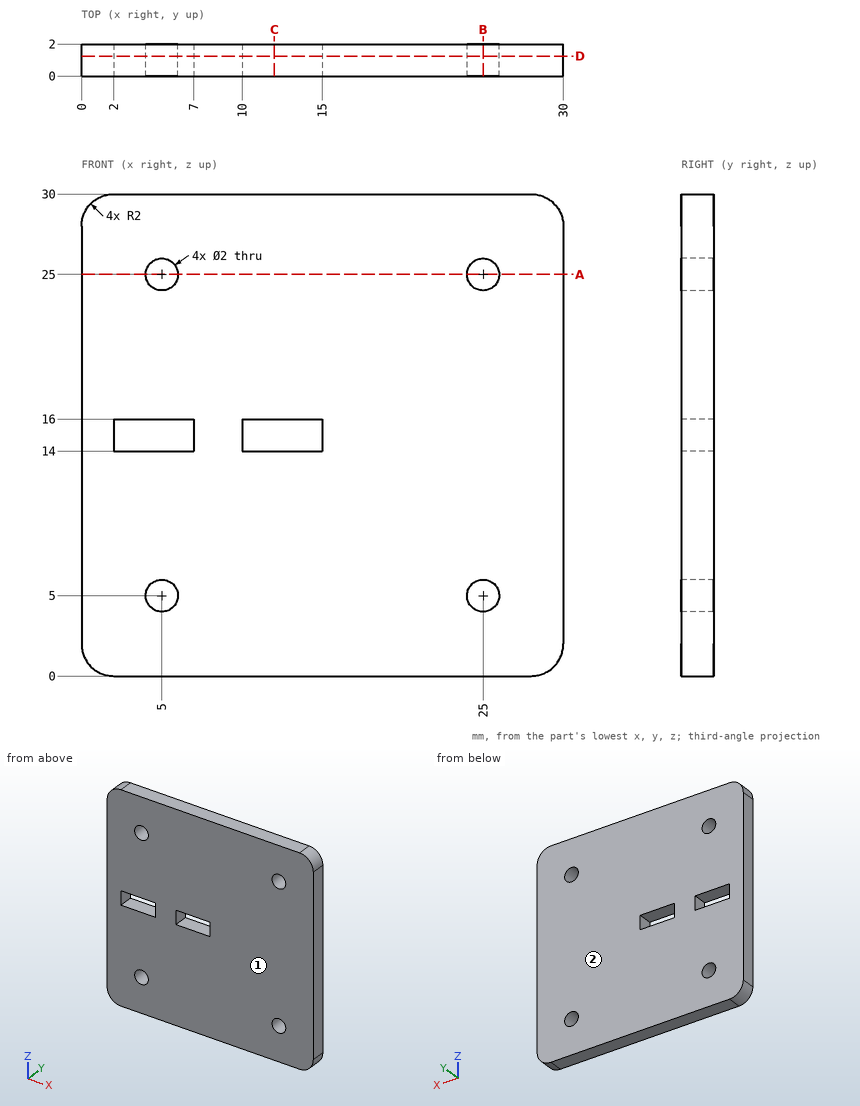
Geometry check sheet. Reference: drawing and pictorial views, mm from the part's lowest x, y, z. Round coordinates to 2 decimals unless told otherwise and drop trailing zeros. Order: outer loops, then holes, each group sorted by start corner. A loop starts at its lowest first (then second) coordinate and runs counter-clockwise, first axis right, second up. Notation, with made-up numbers: M -29.75,-4.5 L 18.25,-4.5 A19 ccw 18.25,15.5 Z; hole C -7,69.25 d1. An arc over 180 degrees is marked long. Answer as CSV lines item,"result".
1) Sectioned sample at A-A on z = 25. Record the cut outline in (x, y).
Entries:
outline,"M 0,0 L 4,0 L 4,2 L 0,2 Z; M 6,0 L 24,0 L 24,2 L 6,2 Z; M 26,0 L 30,0 L 30,2 L 26,2 Z"
2) Sectioned sample at B-B on x = 25. Record the cut outline in (y, z), and give its area (3 significant figures).
Entries:
outline,"M 0,0 L 2,0 L 2,4 L 0,4 Z; M 0,6 L 2,6 L 2,24 L 0,24 Z; M 0,26 L 2,26 L 2,30 L 0,30 Z"
area,"52.0 mm2"
3) Sectioned sample at C-C on x = 12. Record the cut outline in (y, z), and give its area (3 significant figures).
Entries:
outline,"M 0,0 L 2,0 L 2,14 L 0,14 Z; M 0,16 L 2,16 L 2,30 L 0,30 Z"
area,"56.0 mm2"
4) Thickness scan on probe 1 along X at (y, z) = (1.35, 25); probe 2 along X at (y, z) = (0.6, 15); probe 3 along Z at (x, y) = (6.5, 0.8). Record the ranges inside material, lowest first. Write a range as [from, to].
Entries:
probe 1,"[0, 4], [6, 24], [26, 30]"
probe 2,"[0, 2], [7, 10], [15, 30]"
probe 3,"[0, 14], [16, 30]"
5) Gauge pin test, flat ends, axial feed: pin 1 Ø1.5 at (x, z) = (4.5, 3.5) entering from -Y; pin 2 Ø1.8 at (x, z) = (5, 5) entering from +Y. Record the tip position at first contact, or that the pin passes through.
Entries:
pin 1,"y = 0"
pin 2,"through"
6) Mould release check, pull along Y, two halves, no side actions. Record for the marked faces 1 and 2: +Y half, -Y half, draft (parallel to the pull), parting line (faces both ways), or undercut.
Entries:
face 1,"-Y half"
face 2,"+Y half"
7) Sectioned sample at D-D on y = 1.25. Record the cut outline in (x, z).
Entries:
outline,"M 0,2 A2 ccw 2,0 L 28,0 A2 ccw 30,2 L 30,28 A2 ccw 28,30 L 2,30 A2 ccw 0,28 Z; hole M 2,14 L 7,14 L 7,16 L 2,16 Z; hole C 5,5 d2; hole C 5,25 d2; hole M 10,14 L 15,14 L 15,16 L 10,16 Z; hole C 25,5 d2; hole C 25,25 d2"
